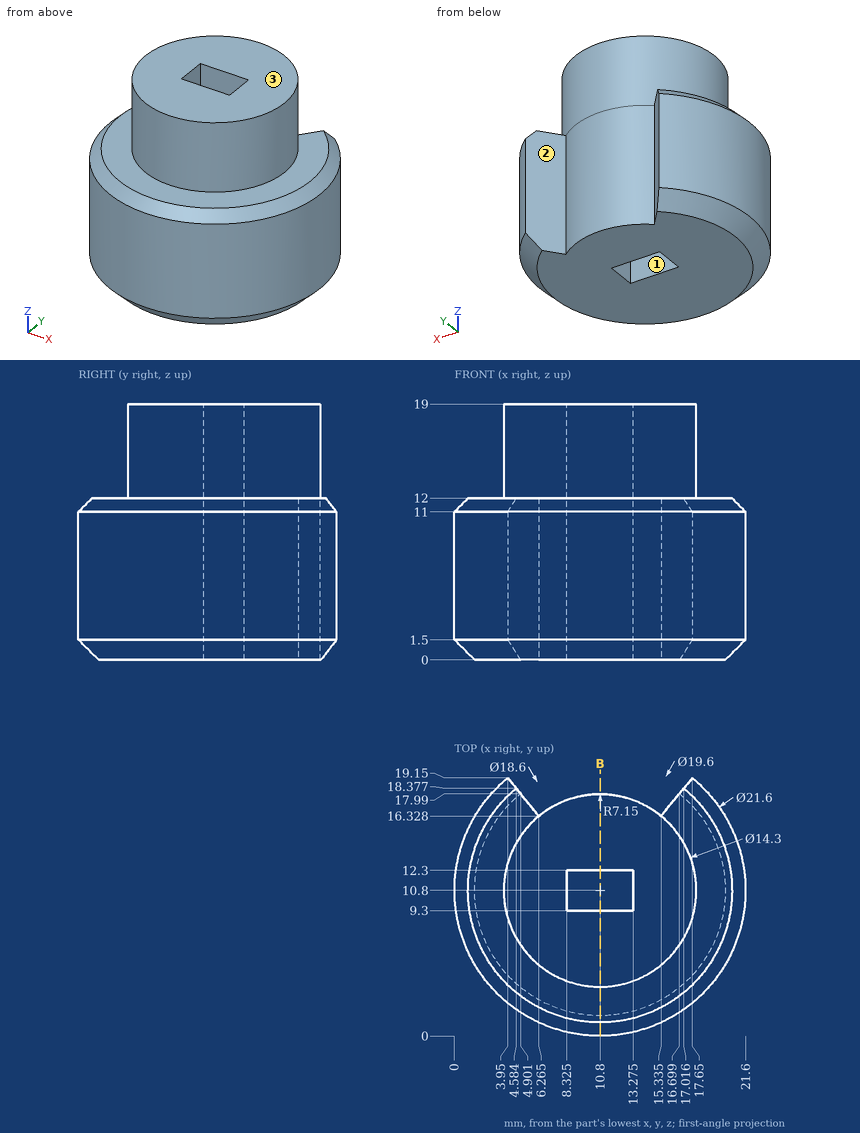
Source: three-view drawing plus pictorial views. Frame: mm from the lowest corner of the part. A direction names the side the tool comes from. Round coordinates to 2 decimals unless told otherwise and drop trailing zeros. Loops run counter-clockwise (first coordinate to the right, second up) from the corner with the lowest first, then second, coordinate; pieces in that order, holes last. Notation, with made-up numbers: M 11.25,61.5 L 69.25,61.5 A20 ccw 69.25,92.5 Z; hole C 9,-4 d5. An arc over 180 degrees is marked long. Put each result on its own line as item: value. Start each with the question number.
(1) Set-up query: the marked faces 1, 2 and 3. Return all of +Z, -Z, +X, -X, +Y, -Y with unobstructed straight access to the full face (end or side cutting, diameter ignored); none if empty.
(2) Contact query for flat-ended pins moving along their axis: pin 1 Ø2 at (x, z) = (11.5, 2) entering from +Y; pin 2 Ø0.9 at (y, z) = (10.5, 14) entering from -X; pin 3 Ø3.5 at (y, z) = (11, 14) entering from +X. Output: stop coordinate, or through.
(3) Section query B-B (x = 10.8). Return loops of the section in (y, z).
(4) Material intervals for line 1 along Y through (x, z) = (8.75, 14.75); line 2 along X through (y, z) = (12.25, 18.25) (1 decimal); line 3 along Z through (x, y) = (19, 10.75), sorted ascending. Write a range as [from, to].
Findings below:
1. face 1: +Z, -Z
1. face 2: +Z, -Z, +Y
1. face 3: +Z, +X, -X, +Y, -Y
2. pin 1: stops at y = 17.95
2. pin 2: stops at x = 3.65
2. pin 3: stops at x = 17.95
3. outline: M 0,1.5 L 1.5,0 L 9.3,0 L 9.3,19 L 3.65,19 L 3.65,12 L 1,12 L 0,11 Z; M 12.3,0 L 17.95,0 L 17.95,19 L 12.3,19 Z
4. line 1: y = [3.95, 9.3], [12.3, 17.65]
4. line 2: x = [3.8, 8.3], [13.3, 17.8]
4. line 3: z = [0, 12]
